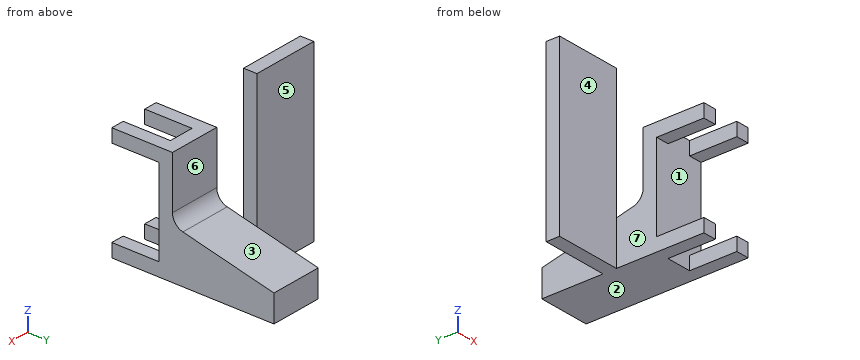
from build123d import *

# Parameters (mm, degrees)
BOSS_EXTRUDE1_DEPTH     = 195
SKETCH2_W               = 645.093387862
SKETCH2_H               = 353.001731878
CUT_EXTRUDE1_DEPTH      = 1
CUT_EXTRUDE1_DEPTH_BACK = 391
FILLET1_R               = 100
SKETCH3_W               = 190
SKETCH3_H               = 353.001731878
CUT_EXTRUDE2_DEPTH      = 1
CUT_EXTRUDE2_DEPTH_BACK = 846.093387862
SKETCH4_W               = 1300
SKETCH4_H               = 100
BOSS_EXTRUDE2_DEPTH     = 500


with BuildPart() as part:
    # Sketch1 → Boss-Extrude1 (new body, symmetric)
    with BuildSketch(Plane(origin=(0, 0, 0), x_dir=(0, 0, -1), z_dir=(1, 0, 0))):
        Polygon((254.379010846, 460.67890474), (81.072942142, -296.617917801), (-389.549913064, -296.617917801), (-389.549913064, -749.619649679), (455.543474798, -749.619649679), (455.543474798, 460.67890474), align=None)
    extrude(amount=BOSS_EXTRUDE1_DEPTH, both=True)

    # Sketch2 → Cut-Extrude1 (cut, two sides)
    with BuildSketch(Plane.ZY.offset(195)) as cut_extrude1_sk:
        with Locations((-32.996780867, -573.11878374)):
            Rectangle(SKETCH2_W, SKETCH2_H)
    extrude(amount=CUT_EXTRUDE1_DEPTH, mode=Mode.SUBTRACT)
    extrude(cut_extrude1_sk.sketch, amount=-CUT_EXTRUDE1_DEPTH_BACK, mode=Mode.SUBTRACT)

    # Fillet1
    fillet1_edges = [part.edges().sort_by_distance(p)[0] for p in [
        (0, -296.617917801, -81.072942142),
    ]]
    fillet(fillet1_edges, radius=FILLET1_R)

    # Sketch3 → Cut-Extrude2 (cut, two sides)
    with BuildSketch(Plane(origin=(0, 0, -455.543474798), x_dir=(-1, 0, 0), z_dir=(0, 0, -1))) as cut_extrude2_sk:
        with Locations((0, -573.11878374)):
            Rectangle(SKETCH3_W, SKETCH3_H)
    extrude(amount=CUT_EXTRUDE2_DEPTH, mode=Mode.SUBTRACT)
    extrude(cut_extrude2_sk.sketch, amount=-CUT_EXTRUDE2_DEPTH_BACK, mode=Mode.SUBTRACT)

    # Sketch4 → Boss-Extrude2 (add)
    with BuildSketch(Plane.ZY.offset(195)):
        with Locations((194.456525202, -46.617917801)):
            Rectangle(SKETCH4_W, SKETCH4_H)
    extrude(amount=BOSS_EXTRUDE2_DEPTH)


solid = part.part
Input: part model. Units: mm. Frame: model coordinates. Face numbers are marked on the shaded views. A direction names the side the tool comes from. Round coordinates to 2 decimals unless told otherwise and drop trailing zeros. Order: outer loops, then holes, each group sorted by start corner. A loop starts at its lowest first (then second) coordinate and runs counter-clockwise, first axis right, second up. Notation, with made-up numbers: (-14, 34.25) - (15, 34.25) arc R22 ccw to (15, 50.25) - close; hole circle Ø7 at (10.5, 30). An arc over 180 degrees is marked (long way). Answer as a JSON object with one key per item and string values. Group by question number.
(1) Cut plane C-C (x = -56). Return loops of the section in (y, z).
(2) Pin query (flat end, axial travel): P1, Ø12, axis at x = -448.5, z = -163.5, coming from the -Y side; P2, Ø8, axis at x = 61.5, z = 57, coming from the -Y side. Return the tip coordinate at first contact, or that it passes through.
(3) Reachability of the marked faces 5, 6 and 7 from +Z, -Z, +X, -X, +Y, -Y: full face, straight path, thin tool, end or side. Return the list, or none.
(4) Cut plane A-A (z = 165.5). Return loops of the section in (x, y).
(5) Material intervals for probe 1 along X at (y, z) = (107.5, -321); probe 2 along Y at (x, z) = (147, 50.5); probe 3 along Y at (x, z) = (-316.5, 210), sorted ascending. Write a range as from..to.
(6) Cut plane D-D (z = -188.5). Return loops of the section in (x, y), then the cut area to 3 significant figures.
(7) Draft query along Z for the marked faces 1, 2, 3 and 4. Return one class per face: released by +Z, released by -Z, zero draft, split by the parting line, or undercut.
(8) Cut plane B-B (y = -444). Return loops of the section in (x, z), then the cut area to 3 significant figures.
Here are the results:
{
 "1": {"outline": "(-396.62, -455.54) - (460.68, -455.54) - (460.68, -254.38) - (-218.93, -98.85) arc R100 cw to (-296.62, -1.37) - (-296.62, 389.55) - (-396.62, 389.55) - close"},
 "2": {"P1": "stops at y = -96.62", "P2": "stops at y = -396.62"},
 "3": {"face 5": "+Z, -Z, -X, +Y", "face 6": "+Z, +X, -X, +Y", "face 7": "+Z, -Z, -X, -Y"},
 "4": {"outline": "(-695, -96.62) - (-195, -96.62) - (-195, 3.38) - (-695, 3.38) - close; (-195, -396.62) - (195, -396.62) - (195, -296.62) - (-195, -296.62) - close"},
 "5": {"probe 1": "x = -195..195", "probe 2": "y = -396.62..-296.62", "probe 3": "y = -96.62..3.38"},
 "6": {"outline": "(-695, -96.62) - (-195, -96.62) - (-195, -396.62) - (195, -396.62) - (195, 172.81) - (-195, 172.81) - (-195, 3.38) - (-695, 3.38) - close", "area": "272,000 mm^2"},
 "7": {"face 1": "undercut", "face 2": "released by -Z", "face 3": "released by +Z", "face 4": "zero draft"},
 "8": {"outline": "(-195, -455.54) - (-95, -455.54) - (-95, -355.54) - (-195, -355.54) - close; (-195, 289.55) - (-95, 289.55) - (-95, 389.55) - (-195, 389.55) - close; (95, -455.54) - (195, -455.54) - (195, -355.54) - (95, -355.54) - close; (95, 289.55) - (195, 289.55) - (195, 389.55) - (95, 389.55) - close", "area": "40,000 mm^2"}
}
